from build123d import *

# Parameters (mm, degrees)
SKETCH1_R                = 15
BOSS_EXTRUDE1_DEPTH      = 5
SKETCH2_R                = 12.6
BOSS_EXTRUDE2_DEPTH      = 10
SKETCH3_R                = 7.5
BOSS_EXTRUDE3_DEPTH      = 5
SKETCH4_R                = 12.625
BOSS_EXTRUDE4_DEPTH      = 10
SKETCH8_R                = 18.75
BOSS_EXTRUDE5_DEPTH      = 5
SKETCH10_R               = 17.5
BOSS_EXTRUDE7_DEPTH      = 10
SKETCH11_R               = 17.65
BOSS_EXTRUDE8_DEPTH      = 10
CUT_EXTRUDE1_REACH       = 63.058
SKETCH12_R               = 1.75
SKETCH12_R_2             = 2.75
CUT_EXTRUDE12_DEPTH      = 53.231456039
CUT_EXTRUDE12_DEPTH_BACK = 53.231456039
SKETCH27_W               = 40.004352786
SKETCH27_H               = 30
BOSS_EXTRUDE11_START     = 2
SKETCH30_R               = 13
SKETCH30_R_2             = 1.75
SKETCH30_R_3             = 2.75
BOSS_EXTRUDE11_DEPTH     = 2
SKETCH31_R               = 1.5
CUT_EXTRUDE13_DEPTH      = 10
SKETCH32_R               = 2.75
CUT_EXTRUDE14_DEPTH      = 4


with BuildPart() as part:
    # Sketch1 → Boss-Extrude1 (new body)
    with BuildSketch(Plane(origin=(0, 0, 0), x_dir=(1, 0, 0), z_dir=(0, 1, 0))):
        with Locations(Location((0, 0, 0), (0, 0, 270))):
            Circle(SKETCH1_R)
    extrude(amount=BOSS_EXTRUDE1_DEPTH)

    # Sketch2 → Boss-Extrude2 (add)
    with BuildSketch(Plane(origin=(0, 5, 0), x_dir=(1, 0, 0), z_dir=(0, 1, 0))):
        with Locations(Location((5, 0, 0), (0, 0, 70.894925587))):
            Circle(SKETCH2_R)
    extrude(amount=BOSS_EXTRUDE2_DEPTH)

    # Sketch3 → Boss-Extrude3 (add)
    with BuildSketch(Plane(origin=(0, 15, 0), x_dir=(1, 0, 0), z_dir=(0, 1, 0))):
        with Locations(Location((0, 0, 0), (0, 0, 270))):
            Circle(SKETCH3_R)
    extrude(amount=BOSS_EXTRUDE3_DEPTH)

    # Sketch4 → Boss-Extrude4 (add)
    with BuildSketch(Plane(origin=(0, 20, 0), x_dir=(1, 0, 0), z_dir=(0, 1, 0))):
        with Locations(Location((-5, 0, 0), (0, 0, 270))):
            Circle(SKETCH4_R)
    extrude(amount=BOSS_EXTRUDE4_DEPTH)

    # Sketch8 → Boss-Extrude5 (add)
    with BuildSketch(Plane(origin=(0, 30, 0), x_dir=(1, 0, 0), z_dir=(0, 1, 0))):
        with Locations(Location((0, 0, 0), (0, 0, 270))):
            Circle(SKETCH8_R)
    extrude(amount=BOSS_EXTRUDE5_DEPTH)

    # Sketch10 → Boss-Extrude7 (add)
    with BuildSketch(Plane(origin=(0, 35, 0), x_dir=(1, 0, 0), z_dir=(0, 1, 0))):
        with Locations(Location((0, 0, 0), (0, 0, 270))):
            Circle(SKETCH10_R)
    extrude(amount=BOSS_EXTRUDE7_DEPTH)

    # Sketch11 → Boss-Extrude8 (add)
    with BuildSketch(Plane.XZ):
        with Locations(Location((0, 0, 0), (0, 0, 270))):
            Circle(SKETCH11_R)
    extrude(amount=BOSS_EXTRUDE8_DEPTH)

    # Cut-Extrude1: up to this face of the body (flat: up to its plane)
    cut_extrude1_end = Plane(part.part.faces().sort_by_distance((0, 45, 0))[0])
    # Sketch12 → Cut-Extrude1 (cut, up to the picked face)
    with BuildSketch(Plane.XZ.offset(10), mode=Mode.PRIVATE) as cut_extrude1_sk1:
        with Locations(Location((0, 6, 0), (0, 0, 270))):
            Circle(SKETCH12_R)
    cut_extrude1_tool1 = split(extrude(cut_extrude1_sk1.sketch, amount=-CUT_EXTRUDE1_REACH, mode=Mode.PRIVATE), bisect_by=cut_extrude1_end, keep=Keep.BOTH, mode=Mode.PRIVATE)
    # Sketch12 → Cut-Extrude1 (cut, up to the picked face)
    with BuildSketch(Plane.XZ.offset(10), mode=Mode.PRIVATE) as cut_extrude1_sk2:
        with Locations(Location((0, -6, 0), (0, 0, 270))):
            Circle(SKETCH12_R)
    cut_extrude1_tool2 = split(extrude(cut_extrude1_sk2.sketch, amount=-CUT_EXTRUDE1_REACH, mode=Mode.PRIVATE), bisect_by=cut_extrude1_end, keep=Keep.BOTH, mode=Mode.PRIVATE)
    # Sketch12 → Cut-Extrude1 (cut, up to the picked face)
    with BuildSketch(Plane.XZ.offset(10), mode=Mode.PRIVATE) as cut_extrude1_sk3:
        with Locations(Location((6, 0, 0), (0, 0, 270))):
            Circle(SKETCH12_R)
    cut_extrude1_tool3 = split(extrude(cut_extrude1_sk3.sketch, amount=-CUT_EXTRUDE1_REACH, mode=Mode.PRIVATE), bisect_by=cut_extrude1_end, keep=Keep.BOTH, mode=Mode.PRIVATE)
    # Sketch12 → Cut-Extrude1 (cut, up to the picked face)
    with BuildSketch(Plane.XZ.offset(10), mode=Mode.PRIVATE) as cut_extrude1_sk4:
        with Locations(Location((-6, 0, 0), (0, 0, 270))):
            Circle(SKETCH12_R)
    cut_extrude1_tool4 = split(extrude(cut_extrude1_sk4.sketch, amount=-CUT_EXTRUDE1_REACH, mode=Mode.PRIVATE), bisect_by=cut_extrude1_end, keep=Keep.BOTH, mode=Mode.PRIVATE)
    # Sketch12 → Cut-Extrude1 (cut, up to the picked face)
    with BuildSketch(Plane.XZ.offset(10), mode=Mode.PRIVATE) as cut_extrude1_sk5:
        with Locations(Location((0, 0, 0), (0, 0, 270))):
            Circle(SKETCH12_R_2)
    cut_extrude1_tool5 = split(extrude(cut_extrude1_sk5.sketch, amount=-CUT_EXTRUDE1_REACH, mode=Mode.PRIVATE), bisect_by=cut_extrude1_end, keep=Keep.BOTH, mode=Mode.PRIVATE)
    add(cut_extrude1_tool1.solids().sort_by(Axis((0, -10, 6), (0, 1, 0)))[0], mode=Mode.SUBTRACT)
    add(cut_extrude1_tool2.solids().sort_by(Axis((0, -10, -6), (0, 1, 0)))[0], mode=Mode.SUBTRACT)
    add(cut_extrude1_tool3.solids().sort_by(Axis((6, -10, 0), (0, 1, 0)))[0], mode=Mode.SUBTRACT)
    add(cut_extrude1_tool4.solids().sort_by(Axis((-6, -10, 0), (0, 1, 0)))[0], mode=Mode.SUBTRACT)
    add(cut_extrude1_tool5.solids().sort_by(Axis((0, -10, 0), (0, 1, 0)))[0], mode=Mode.SUBTRACT)

    # Sketch27 → Cut-Extrude12 (cut, two sides: drawn at the far end of the back side and taken through both)
    with BuildSketch(Plane(origin=(0, 0, 0), x_dir=(0, 0, -1), z_dir=(1, 0, 0)).offset(-CUT_EXTRUDE12_DEPTH_BACK)):
        with Locations((-0.026275673, 5)):
            Rectangle(SKETCH27_W, SKETCH27_H)
    extrude(amount=CUT_EXTRUDE12_DEPTH + CUT_EXTRUDE12_DEPTH_BACK, mode=Mode.SUBTRACT)

    # Sketch30 → Boss-Extrude11 (add)
    with BuildSketch(Plane.XZ.offset(-30).offset(BOSS_EXTRUDE11_START)):
        with Locations(Location((-5, 0, 0), (0, 0, 90))):
            Circle(SKETCH30_R)
        with Locations(Location((0, -6, 0), (0, 0, 90))):
            Circle(SKETCH30_R_2, mode=Mode.SUBTRACT)
        with Locations(Location((-6, 0, 0), (0, 0, 90))):
            Circle(SKETCH30_R_2, mode=Mode.SUBTRACT)
        with Locations(Location((0, 6, 0), (0, 0, 90))):
            Circle(SKETCH30_R_2, mode=Mode.SUBTRACT)
        with Locations(Location((6, 0, 0), (0, 0, 336.579668072))):
            Circle(SKETCH30_R_2, mode=Mode.SUBTRACT)
        with Locations(Location((0, 0, 0), (0, 0, 90))):
            Circle(SKETCH30_R_3, mode=Mode.SUBTRACT)
    extrude(amount=-BOSS_EXTRUDE11_DEPTH)

    # Sketch31 → Cut-Extrude13 (cut)
    with BuildSketch(Plane(origin=(0, 45, 0), x_dir=(1, 0, 0), z_dir=(0, 1, 0))):
        with Locations(Location((-7.424621202, 7.424621202, 0), (0, 0, 270))):
            Circle(SKETCH31_R)
        with Locations(Location((7.424621202, 7.424621202, 0), (0, 0, 270))):
            Circle(SKETCH31_R)
        with Locations(Location((7.424621202, -7.424621202, 0), (0, 0, 270))):
            Circle(SKETCH31_R)
        with Locations(Location((-7.424621202, -7.424621202, 0), (0, 0, 270))):
            Circle(SKETCH31_R)
    extrude(amount=-CUT_EXTRUDE13_DEPTH, mode=Mode.SUBTRACT)

    # Sketch32 → Cut-Extrude14 (cut)
    with BuildSketch(Plane(origin=(0, 45, 0), x_dir=(1, 0, 0), z_dir=(0, 1, 0))):
        with Locations(Location((-6, 0, 0), (0, 0, 270))):
            Circle(SKETCH32_R)
        with Locations(Location((0, 6, 0), (0, 0, 270))):
            Circle(SKETCH32_R)
        with Locations(Location((6, 0, 0), (0, 0, 270))):
            Circle(SKETCH32_R)
        with Locations(Location((0, -6, 0), (0, 0, 270))):
            Circle(SKETCH32_R)
    extrude(amount=-CUT_EXTRUDE14_DEPTH, mode=Mode.SUBTRACT)


solid = part.part
Geometry: final body of the model. Coordinates: model frame, mm. A direction names the side the tool comes from. Round coordinates to 2 decimals unless told otherwise and drop trailing zeros. Write each loop counter-clockwise with the first axis right and the second up, starting at its lowest first coordinate (ties: lowest second). Pieces come first, ordered by that corner, then holes. Notation, with made-up numbers: M 86.5,-39.5 L 113.5,-39.5 A19 ccw 113.5,-26.5 Z; hole C 71,72 d1. An arc over 180 degrees is marked long. Write item = value, one per line.
Item 1: Material intervals for line 1 along X through (y, z) = (41.95, 0); line 2 along X through (y, z) = (22.25, 0) (3 decimals); line 3 along X through (y, z) = (42.25, -7), sorted ascending. Write a range as [from, to].
Findings:
line_1 = [-17.5, -8.75], [-3.25, -2.75], [2.75, 3.25], [8.75, 17.5]
line_2 = [-17.625, -7.75], [-4.25, -2.75], [2.75, 4.25]
line_3 = [-16.04, -8.86], [-5.99, -2.56], [2.56, 5.99], [8.86, 16.04]
Item 2: Pin query (flat end, axial travel): P1, Ø4.5, axis at x = -6, z = 0, coming from the +Y side; P2, Ø7, axis at x = -6, z = 0, coming from the -Y side; P3, Ø6, axis at y = 30, z = -2.5, coming from the +X side; P4, Ø2.5, axis at x = -7.5, z = -7.5, coming from the +Y side. Return the tip coordinate at first contact, or that it passes through.
Findings:
P1 = 41
P2 = 20
P3 = 18.75
P4 = 35
Item 3: Section query A-A on z = 0. State how many separate pieces and enclosed holes the cut face has, then the cut area to 3 significant figures.
Findings:
separate_pieces = 4
enclosed_holes = 0
area = 464 mm^2
Item 4: Pull-direction query (X, two-part tool) for faces 1 (the face through (-10.648, 39.93, -13.887)), 2 (the face through (-1.05, 43.03, -3.46)), 3 (the face through (-4, 45, 4)); classes: pulls with the +X half, pulls with the -X half, needs draft (parallel to the pull), parting line crosses it, or undercut.
Findings:
face_1 = parting line crosses it
face_2 = undercut
face_3 = needs draft
Item 5: Section query B-B on y = 33.75. Return loops of the section in (x, z).
Findings:
outline = C 0,0 d37.5; hole C -6,0 d3.5; hole C 0,0 d5.5; hole C 0,-6 d3.5; hole C 0,6 d3.5; hole C 6,0 d3.5
Item 6: Access query for faces 4 (the face through (-5.937, 40.07, -7.62)), 5 (the face through (-11.41, 32.47, -14.88)), 6 (the face through (9, 30, 0)). Directions: +Z, -Z, +X, -X, +Y, -Y. A direction counts if a zero-diameter tool reaches every point of the face in a straight line with its end or side. Return the directions, or none.
Findings:
face_4 = +Y
face_5 = +Y, -Y
face_6 = -Y
Item 7: Section query C-C on x = -11.5. Return loops of the section in (y, z).
Findings:
outline = M 20,-10.82 L 28,-10.82 L 28,-11.26 L 30,-11.26 L 30,-14.81 L 35,-14.81 L 35,-13.19 L 45,-13.19 L 45,13.19 L 35,13.19 L 35,14.81 L 30,14.81 L 30,11.26 L 28,11.26 L 28,10.82 L 20,10.82 Z
